Can you work these out from the model? Positions are in its coordinate system, mm. Coordinates: 2 decimals unless noted, no trailing zeros. Order: outer loops, then holes, each group sorted by start corner. A loop starts at its lowest first (then second) coordinate and runs counter-clockwise, first axis right, second up. Notation, with made-up numbers: (48, 44) -> (55, 44) arc R23 ccw to (55, 83) -> close; hole circle Ø7 at (-25.5, 50). An arc over 180 degrees is marked (long way). Answer in a Markdown table with one row per item.
Autodesk Inventor part; units mm, degrees
ref_plane "YZ Plane" through (0, 0, 0) normal (1, 0, 0) x (0, 1, 0)
ref_plane "XZ Plane" through (0, 0, 0) normal (0, 1, 0) x (-1, 0, 0)
ref_plane "XY Plane" through (0, 0, 0) normal (0, 0, 1) x (1, 0, 0)
sketch "Sketch1" plane through (0, 0, 0) normal (0, 0, 1) x (1, 0, 0)
  point P0 (0, 0)
sketch "Sketch2" plane through (0, 0, 0) normal (0, 0, 1) x (1, 0, 0)
  line L0 (0, 0) -> (335, 0)
  line L1 (335, 0) -> (335, 450)
  line L2 (335, 450) -> (0, 450)
  line L3 (0, 450) -> (0, 0)
  line L4 (0, 0) -> (167.5, 0)
  dimension "d0" = 335
  dimension "d1" = 450
  dimension "d2" = 167.5
extrude "Extrusion1" add sketch "Sketch2" along normal blind 7
sketch "Sketch3" plane through (0, 0, 7) normal (0, 0, 1) x (1, 0, 0)
  line L0 (0, 0) -> (167.5, 0)
  line L1 (0, 0) -> (335, 0)
  line L2 (167.5, 0) -> (167.5, 450)
  line L3 (335, 450) -> (0, 450)
  line L4 (0, 0) -> (0, 325)
  line L5 (0, 450) -> (0, 0)
  line L6 (0, 325) -> (335, 325)
  line L7 (335, 0) -> (335, 450)
  line L8 (335, 325) -> (167.5, 450)
  line L9 (167.5, 450) -> (0, 325)
  dimension "d5" = 167.5
  dimension "d6" = 325
extrude "Extrusion2" cut sketch "Sketch3" against normal blind 166.0375 contours L5 L3 L9
sketch "Sketch5" plane through (0, 0, 7) normal (0, 0, 1) x (1, 0, 0)
  line L0 (167.5, 450) -> (335, 450)
  line L1 (335, 450) -> (167.5, 450)
  line L2 (335, 450) -> (335, 0)
  line L3 (335, 0) -> (335, 450)
  line L4 (335, 0) -> (335, 325)
  line L5 (167.5, 450) -> (335, 325)
  line L6 (335, 450) -> (167.5, 450)
  line L7 (335, 325) -> (335, 450)
  point P0 (0, 0)
  dimension "d10" = 325
extrude "Extrusion3" cut sketch "Sketch5" against normal blind 305.45
sketch "Sketch6" plane through (0, 0, 7) normal (0, 0, 1) x (1, 0, 0)
  point P0 (0, 0)
sketch "Sketch7" plane through (0, 0, 7) normal (0, 0, 1) x (1, 0, 0)
  point P0 (0, 0)
sketch "Sketch8" plane through (0, 0, 7) normal (0, 0, 1) x (1, 0, 0)
  point P0 (0, 0)
sketch "Sketch9" plane through (0, 0, 7) normal (0, 0, 1) x (1, 0, 0)
  point P0 (0, 0)
sketch "Sketch12" plane through (0, 0, 7) normal (0, 0, 1) x (1, 0, 0)
  line L0 (207.5, 195) -> (127.5, 195)
  line L1 (167.5, 0) -> (207.5, 0)
  line L2 (0, 0) -> (335, 0)
  line L3 (207.5, 0) -> (127.5, 0)
  line L4 (207.5, 0) -> (207.5, 130)
  line L5 (127.5, 0) -> (207.5, 0)
  line L6 (207.5, 0) -> (207.5, 130)
  line L7 (207.5, 130) -> (127.5, 130)
  line L8 (127.5, 130) -> (127.5, 0)
  dimension "d25" = 40
  dimension "d26" = 80
  dimension "d27" = 130
extrude "Extrusion6" cut sketch "Sketch12" against normal blind 10
sketch "Sketch13" plane through (0, 0, 7) normal (0, 0, 1) x (1, 0, 0)
  line L0 (167.5, 450) -> (167.5, 0)
  line L1 (0, 0) -> (127.5, 0)
  line L2 (0, 325) -> (335, 325)
  line L3 (335, 0) -> (335, 325)
  line L4 (127.5, 130) -> (207.5, 130)
  line L5 (167.5, 130) -> (167.5, 195)
  line L6 (167.5, 195) -> (167.5, 235.5)
  line L7 (167.5, 235.5) -> (167.5, 276)
  circle A0 centre (167.5, 235.5) radius 40.5
  dimension "d30" = 65
  dimension "d31" = 40.5
  dimension "d32" = 40.5
extrude "Extrusion7" cut sketch "Sketch13" against normal blind 10
sketch "Sketch18" plane through (0, 0, 7) normal (0, 0, 1) x (1, 0, 0)
  line L0 (0, 0) -> (335, 0)
  line L1 (335, 0) -> (335, 130)
  line L2 (335, 130) -> (0, 130)
  line L3 (0, 130) -> (0, 0)
  dimension "d43" = 335
  dimension "d44" = 130
extrude "Extrusion10" cut sketch "Sketch18" against normal blind 10
properties part number "frente"
(1) Suppose I cut it at C-C (z = 3). Please give me the cut outline in (x, y).
Response values:
| item | result |
|---|---|
| outline | (0, 130) -> (335, 130) -> (335, 325) -> (167.5, 450) -> (0, 325) -> close; hole circle Ø81 at (167.5, 235.5) |
(2) I need wall thicknesses on line 1 (X direction, y = 235.5, z = 2); line 2 (Y direction, x = 167.5, z = 3.5); line 3 (Y direction, x = 154.5, z = 5). Which ranges of each line are inside material? Lowest first, please. Write a range as [from, to].
Response values:
| item | result |
|---|---|
| line 1 | [0, 127], [208, 335] |
| line 2 | [130, 195], [276, 450] |
| line 3 | [130, 197.14], [273.86, 440.3] |
(3) Suppose I cut it at B-B (x = 196.5). Please give me the cut outline in (y, z).
Response values:
| item | result |
|---|---|
| outline | (130, 0) -> (207.23, 0) -> (207.23, 7) -> (130, 7) -> close; (263.77, 0) -> (428.36, 0) -> (428.36, 7) -> (263.77, 7) -> close |
(4) Will these pins go through, and if not, where does the flat tip stop? pin 1 Ø1 at (x, z) = (286, 3.5) entering from +Y; pin 2 Ø1.5 at (x, z) = (120.5, 3.5) entering from +Y.
Response values:
| item | result |
|---|---|
| pin 1 | y = 361.94 |
| pin 2 | y = 415.49 |
(5) Suppose I cut it at A-A (y = 235.5). Please give me the cut outline in (x, z).
Response values:
| item | result |
|---|---|
| outline | (0, 0) -> (127, 0) -> (127, 7) -> (0, 7) -> close; (208, 0) -> (335, 0) -> (335, 7) -> (208, 7) -> close |
(6) Suppose I cut it at D-D (y = 430). Please give me the cut outline in (x, z), and give its area (3 significant figures).
Response values:
| item | result |
|---|---|
| outline | (140.7, 0) -> (194.3, 0) -> (194.3, 7) -> (140.7, 7) -> close |
| area | 375 mm2 |
